from build123d import *

# Parameters (mm, degrees)
SKETCH1_R           = 2.2
BOSS_EXTRUDE1_DEPTH = 3.9
THREAD1_PITCH       = 0.8
CHAMFER1_SIZE       = 0.5


with BuildPart() as part:
    # Sketch1 → Boss-Extrude1 (new body)
    with BuildSketch(Plane(origin=(0, 0, 0), x_dir=(1, 0, 0), z_dir=(0, 1, 0))):
        Polygon((0, -4.474464586), (3.875, -2.237232293), (3.875, 2.237232293), (0, 4.474464586), (-3.875, 2.237232293), (-3.875, -2.237232293), align=None)
        with Locations(Location((0, 0, 0), (0, 0, 270))):
            Circle(SKETCH1_R, mode=Mode.SUBTRACT)
    extrude(amount=BOSS_EXTRUDE1_DEPTH)

    # Thread1: the profile of Thread Profile1 profile screwed along a right-hand helix of 5.625 turns, 8 arcs to a turn; built about Z, then put on its axis
    thread1_z = Axis((0, 0, 0), (0, 0, 1))
    thread1_corners = [(2.1997, 0, -0.000173205), (2.6330127, 0, 0.249999999), (2.6330127, 0, 0.349999999), (2.1997, 0, 0.600173203)]
    with BuildLine(mode=Mode.PRIVATE) as thread1_profile:
        Line(thread1_corners[0], thread1_corners[1])
        Line(thread1_corners[1], thread1_corners[2])
        Line(thread1_corners[2], thread1_corners[3])
        Line(thread1_corners[3], thread1_corners[0])
    thread1_cap = Face(thread1_profile.wire())
    thread1_turn_angles = [0, 22.5, 45, 67.5, 90, 112.5, 135, 157.5, 180, 202.5, 225, 247.5, 270, 292.5, 315, 337.5, 360]
    thread1_turn_weights = [1, 0.9238795325112867, 1, 0.9238795325112867, 1, 0.9238795325112867, 1, 0.9238795325112867, 1, 0.9238795325112867, 1, 0.9238795325112867, 1, 0.9238795325112867, 1, 0.9238795325112867, 1]
    thread1_turn_rails = [Edge.make_bspline([Vector(p[0], p[1], 0).rotate(thread1_z, thread1_turn_angles[k]) / thread1_turn_weights[k] + Vector(0, 0, p[2] + THREAD1_PITCH * thread1_turn_angles[k] / 360) for k in range(17)], [0, 0, 0, 1, 1, 2, 2, 3, 3, 4, 4, 5, 5, 6, 6, 7, 7, 8, 8, 8], 2, thread1_turn_weights) for p in thread1_corners]
    thread1_turn_sides = [Face.make_surface_from_curves(thread1_turn_rails[p[0]], thread1_turn_rails[p[1]]) for p in [(0, 1), (1, 2), (2, 3), (3, 0)]]
    thread1_last_angles = [1800, 1822.5, 1845, 1867.5, 1890, 1912.5, 1935, 1957.5, 1980, 2002.5, 2025]
    thread1_last_weights = [1, 0.9238795325112867, 1, 0.9238795325112867, 1, 0.9238795325112867, 1, 0.9238795325112867, 1, 0.9238795325112867, 1]
    thread1_last_rails = [Edge.make_bspline([Vector(p[0], p[1], 0).rotate(thread1_z, thread1_last_angles[k]) / thread1_last_weights[k] + Vector(0, 0, p[2] + THREAD1_PITCH * thread1_last_angles[k] / 360) for k in range(11)], [0, 0, 0, 1, 1, 2, 2, 3, 3, 4, 4, 5, 5, 5], 2, thread1_last_weights) for p in thread1_corners]
    thread1_last_sides = [Face.make_surface_from_curves(thread1_last_rails[p[0]], thread1_last_rails[p[1]]) for p in [(0, 1), (1, 2), (2, 3), (3, 0)]]
    thread1 = Plane(origin=(0, 4.5, 0), x_dir=(-1, 0, 0), z_dir=(0, -1, 0)) * Solid(Shell([*[p.moved(Location((0, 0, THREAD1_PITCH * i))) for i in range(5) for p in thread1_turn_sides], *thread1_last_sides, thread1_cap, thread1_cap.rotate(thread1_z, 2025).moved(Location((0, 0, THREAD1_PITCH * 2025 / 360)))]))
    add(thread1, mode=Mode.SUBTRACT)

    # Chamfer1
    chamfer1_edges = [part.edges().sort_by_distance(p)[0] for p in [
        (3.875, 3.9, 0),
        (1.9375, 3.9, -3.35584844),
        (-1.9375, 3.9, -3.35584844),
        (-3.875, 3.9, 0),
        (-1.9375, 3.9, 3.35584844),
        (-3.875, 0, 0),
        (-1.9375, 0, -3.35584844),
        (1.9375, 0, -3.35584844),
        (1.9375, 3.9, 3.35584844),
        (3.875, 0, 0),
        (1.9375, 0, 3.35584844),
        (-1.9375, 0, 3.35584844),
    ]]
    chamfer(chamfer1_edges, length=CHAMFER1_SIZE)


solid = part.part
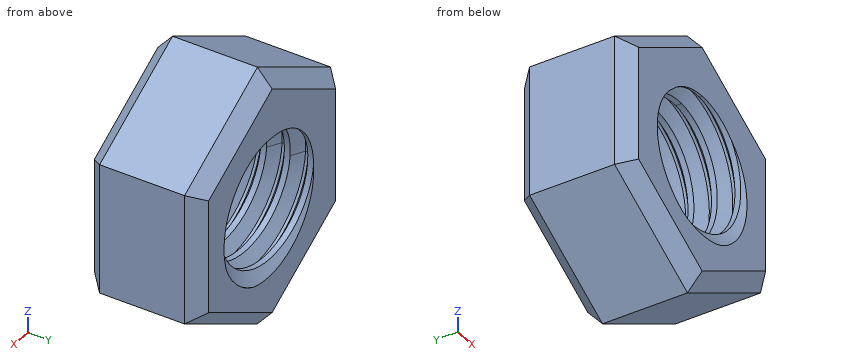
The model under review builds one solid part; all positions refer to its coordinate system, in mm. Coordinates: 2 decimals unless noted, no trailing zeros. Loops run counter-clockwise (first coordinate to the right, second up) from the corner with the lowest first, then second, coordinate; pieces in that order, holes last. Notation, with made-up numbers: (24, -21) -> (74, -21) arc R12 cw to (74, -2) -> close; hole circle Ø7 at (57, 54). An arc over 180 degrees is marked (long way). Use a Markdown table: item, result. Add a question column.
1. Add section A-A on x = -3. Write out the cut boundary in (y, z).
2. To check wall thickness, follow line 1 (Y direction, x = 2.25, z = 0.25); line 2 (Y direction, x = 2.25, z = 0.75); line 3 (Z direction, x = 0.25, y = 0.25). State the ranges of each line that lie inside material, in increasing order.
3. Clearance check with flat-ended pins moving along their axes: pin 1 Ø1.5 at (x, y) = (-2, 3) entering from +Z; pin 2 Ø3.5 at (x, z) = (0, 0) entering from +Y; pin 3 Ø2 at (x, y) = (-3, 1.5) entering from -Z. State where each tip first meets the part, or that it passes through.
4. Add section B-B on z = 2.5. Give the number of separate pieces and of enclosed holes in the cut face, plus the area to 3 significant figures.
Returned:
| question | item | result |
|---|---|---|
| 1 | outline | (0, -2.17) -> (0.5, -2.74) -> (3.4, -2.74) -> (3.9, -2.17) -> (3.9, 2.17) -> (3.4, 2.74) -> (0.5, 2.74) -> (0, 2.17) -> close |
| 2 | line 1 | y = 0.05 to 0.32, 0.85 to 1.12, 1.65 to 1.92, 2.45 to 2.72, 3.25 to 3.52 |
| 2 | line 2 | y = 0 to 0.36, 0.76 to 1.16, 1.56 to 1.96, 2.36 to 2.76, 3.16 to 3.56 |
| 2 | line 3 | z = -4.04 to -2.25, 2.43 to 4.04 |
| 3 | pin 1 | stops at z = 3.75 |
| 3 | pin 2 | passes through |
| 3 | pin 3 | stops at z = -3.32 |
| 4 | separate pieces | 1 |
| 4 | enclosed holes | 5 |
| 4 | area | 24.0 mm² |
